from build123d import *

# Parameters (mm, degrees)
SKETCH1_R           = 15
BOSS_EXTRUDE1_DEPTH = 20
SKETCH2_R           = 10
CUT_EXTRUDE1_DEPTH  = 10
CUT_EXTRUDE3_START  = -2
SKETCH3_R           = 10
CUT_EXTRUDE3_DEPTH  = 2
SKETCH4_R           = 2
BOSS_EXTRUDE2_DEPTH = 5
BOSS_EXTRUDE3_START = 2
SKETCH5_R           = 2
BOSS_EXTRUDE3_DEPTH = 2
FILLET2_R           = 2.5
FILLET3_R           = 2.5


with BuildPart() as part:
    # Sketch1 → Boss-Extrude1 (new body)
    with BuildSketch(Plane.XY):
        Circle(SKETCH1_R)
    extrude(amount=BOSS_EXTRUDE1_DEPTH)

    # Sketch2 → Cut-Extrude1 (cut)
    with BuildSketch(Plane.XY.offset(20)):
        Circle(SKETCH2_R)
    extrude(amount=-CUT_EXTRUDE1_DEPTH, mode=Mode.SUBTRACT)

    # Sketch3 → Cut-Extrude3 (cut)
    with BuildSketch(Plane(origin=(0, 0, 0), x_dir=(-1, 0, 0), z_dir=(0, 0, -1)).offset(CUT_EXTRUDE3_START)):
        with Locations(Location((0, 0, 0), (0, 0, 180))):
            Circle(SKETCH3_R)
    extrude(amount=CUT_EXTRUDE3_DEPTH, mode=Mode.SUBTRACT)

    # Sketch4 → Boss-Extrude2 (add)
    with BuildSketch(Plane.XY.offset(10)):
        Circle(SKETCH4_R)
    extrude(amount=BOSS_EXTRUDE2_DEPTH)

    # Sketch5 → Boss-Extrude3 (add)
    with BuildSketch(Plane(origin=(0, 0, 2), x_dir=(-1, 0, 0), z_dir=(0, 0, -1)).offset(BOSS_EXTRUDE3_START)):
        with Locations(Location((0, 0, 0), (0, 0, 180))):
            Circle(SKETCH5_R)
    extrude(amount=-BOSS_EXTRUDE3_DEPTH)

    # Fillet2
    fillet2_edges = [part.edges().sort_by_distance(p)[0] for p in [
        (-15, 0, 20),
    ]]
    fillet(fillet2_edges, radius=FILLET2_R)

    # Fillet3
    fillet3_edges = [part.edges().sort_by_distance(p)[0] for p in [
        (-15, 0, 0),
    ]]
    fillet(fillet3_edges, radius=FILLET3_R)


solid = part.part
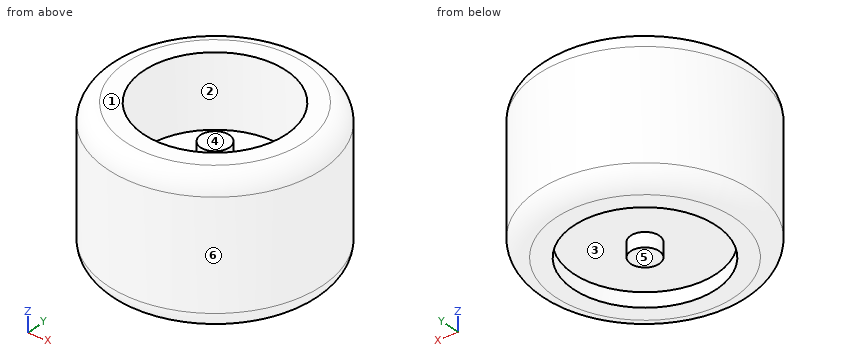
Geometry check sheet. Reference: the model listing, model coordinates, mm. Face numbers are marked on the shaded views. A direction names the side the tool comes from. Round coordinates to 2 decimals unless told otherwise and drop trailing zeros. Write each loop counter-clockwise with the first axis right and the second up, starting at its lowest first coordinate (ties: lowest second). Pieces come first, ordered by that corner, then holes.
Item 1: Section check B-B (z = 14). Record the boundary of the cut face in (x, y), plus the area to 3 significant figures.
Determined:
outline: circle Ø30 at (0, 0); circle Ø4 at (0, 0); hole circle Ø20 at (0, 0)
area: 405 mm2
Item 2: Section check D-D (z = 16.75). Record the boundary of the cut face in (x, y).
Determined:
outline: circle Ø30 at (0, 0); hole circle Ø20 at (0, 0)
Item 3: Access from +Z, -Z, +X, -X, +Y, -Y to the whole of each face (thin tool, end or side, straight path). Record for the marked faces 1, 2 and 3.
Determined:
face 1: +Z, +X, -X, +Y, -Y
face 2: +Z
face 3: -Z
Item 4: Go/stop test with flat-tipped pins: pin 1 Ø6 at (x, z) = (-5.5, 5.5) entering from -Y; pin 2 Ø1.2 at (x, y) = (0.5, 0) entering from +Z; pin 3 Ø1.5 at (y, z) = (11, 15.5) entering from +X. Record where each tip stops, or that it passes through.
Determined:
pin 1: stops at y = -14.79
pin 2: stops at z = 15
pin 3: stops at x = 10.95
Item 5: Material ranges on line 1 along Y through (x, z) = (0, 1.3); line 2 along Z through (x, y) = (2, 7.25); line 3 along X through (y, z) = (1.75, 1), recorded low to high.
Determined:
line 1: y = -14.69 to -10, -2 to 2, 10 to 14.69
line 2: z = 2 to 10
line 3: x = -14.39 to -9.85, -0.97 to 0.97, 9.85 to 14.39
Item 6: Section check A-A (y = 0). Record the boundary of the cut face in (x, z).
Determined:
outline: (-15, 2.5) arc R2.5 ccw to (-12.5, 0) - (-10, 0) - (-10, 2) - (-2, 2) - (-2, 0) - (2, 0) - (2, 2) - (10, 2) - (10, 0) - (12.5, 0) arc R2.5 ccw to (15, 2.5) - (15, 17.5) arc R2.5 ccw to (12.5, 20) - (10, 20) - (10, 10) - (2, 10) - (2, 15) - (-2, 15) - (-2, 10) - (-10, 10) - (-10, 20) - (-12.5, 20) arc R2.5 ccw to (-15, 17.5) - close
Item 7: Mould release check, pull along X, two halves, no side actions. Record for the marked faces 4, 5 and 6: +X half, -X half, draft (parallel to the pull), parting line (faces both ways), or undercut.
Determined:
face 4: undercut
face 5: draft
face 6: parting line
